```python
from build123d import *

# Parameters (mm, degrees)
SKETCH1_W           = 45.5
SKETCH1_H           = 37
BASIS_DEPTH         = 4
CUT_EXTRUDE10_DEPTH = 0.1
CUT_EXTRUDE14_DEPTH = 0.1
SKETCH10_9_R        = 5.5
SKETCH10_9_R_2      = 5.3
CUT_EXTRUDE16_DEPTH = 0.1
FILLET1_R           = 0.2


with BuildPart() as part:
    # Sketch1 → Basis (new body)
    with BuildSketch(Plane.XY):
        with Locations((22.75, 18.5)):
            Rectangle(SKETCH1_W, SKETCH1_H)
        Polygon((14.5, 39.5), (12.5, 37), (16.5, 37), align=None)
        Polygon((31, 39.5), (29, 37), (33, 37), align=None)
        Polygon((16.5, 0), (12.5, 0), (14.5, -2.5), align=None)
        Polygon((33, 0), (29, 0), (31, -2.5), align=None)
    extrude(amount=BASIS_DEPTH)

    # Sketch10 → Cut-Extrude10 (cut)
    with BuildSketch(Plane.XY.offset(4)):
        with BuildLine():
            Line((10.75, 12), (34.75, 12))
            add(Edge.make_bspline(
                [(10.75, 12), (10.75, 5), (22.75, 5), (34.75, 5), (34.75, 12)],
                knots=[0, 0, 0, 1.570796327, 1.570796327, 3.141592654, 3.141592654, 3.141592654], degree=2, weights=[1, 0.707106781, 1, 0.707106781, 1]))
        make_face()
        with BuildLine():
            Line((10.955151261, 11.8), (34.544848739, 11.8))
            add(Edge.make_bspline(
                [(34.544848739, 11.8), (34.522497462, 11.366189062), (34.337619942, 10.522792028), (33.405825268, 8.867470761), (31.220098023, 7.030241966), (27.326621533, 5.547133455), (22.75, 5.026433272), (18.173378467, 5.547133455), (14.279901977, 7.030241966), (12.094174732, 8.867470761), (11.162380058, 10.522792028), (10.977502538, 11.366189062), (10.955151261, 11.8)],
                knots=[3.171638741, 3.171638741, 3.171638741, 3.171638741, 3.364232521, 3.556826301, 3.942013861, 4.32720142, 4.71238898, 5.09757654, 5.4827641, 5.86795166, 6.06054544, 6.25313922, 6.25313922, 6.25313922, 6.25313922], degree=3))
        make_face(mode=Mode.SUBTRACT)
    extrude(amount=-CUT_EXTRUDE10_DEPTH, mode=Mode.SUBTRACT)

    # Sketch10_6 → Cut-Extrude14 (cut)
    with BuildSketch(Plane.XY.offset(4)):
        with BuildLine():
            ThreePointArc((12.125360528, 18.820696373), (13.25, 18.7), (14.374639472, 18.820696373))
            add(Edge.make_bspline(
                [(14.374639472, 18.820696373), (17.140586708, 20.492548158), (15.195293354, 23.38435682), (13.25, 26.276165482), (11.304706646, 23.38435682), (9.359413292, 20.492548158), (12.125360528, 18.820696373)],
                knots=[0.46660386, 0.46660386, 0.46660386, 2.249929722, 2.249929722, 4.033255585, 4.033255585, 5.816581447, 5.816581447, 5.816581447], degree=2, weights=[1, 0.62811894, 1, 0.62811894, 1, 0.62811894, 1]))
        make_face()
    cut_extrude14 = extrude(amount=-CUT_EXTRUDE14_DEPTH, mode=Mode.SUBTRACT)

    # Sketch10_9 → Cut-Extrude16 (cut)
    with BuildSketch(Plane.XY.offset(4)):
        with Locations((13.25, 24)):
            Circle(SKETCH10_9_R)
        with Locations((13.25, 24)):
            Circle(SKETCH10_9_R_2, mode=Mode.SUBTRACT)
    cut_extrude16 = extrude(amount=-CUT_EXTRUDE16_DEPTH, mode=Mode.SUBTRACT)

    # Mirror1: Cut-Extrude14, Cut-Extrude16 across plane
    add(cut_extrude14.mirror(Plane.ZY.offset(-22.75)), mode=Mode.SUBTRACT)
    add(cut_extrude16.mirror(Plane.ZY.offset(-22.75)), mode=Mode.SUBTRACT)

    # Fillet1
    fillet1_edges = [part.edges().sort_by_distance(p)[0] for p in [
        (10.955151261, 11.8, 3.95),
        (34.544848739, 11.8, 3.95),
        (10.75, 12, 3.95),
        (34.75, 12, 3.95),
    ]]
    fillet(fillet1_edges, radius=FILLET1_R)


solid = part.part
```
Input: part model. Units: mm. Frame: model coordinates. A direction names the side the tool comes from. Coordinates: 2 decimals unless noted, no trailing zeros. Loops run counter-clockwise (first coordinate to the right, second up) from the corner with the lowest first, then second, coordinate; pieces in that order, holes last. Notation, with made-up numbers: (44, -15.5) -> (64, -15.5) arc R21 cw to (64, 6.5) -> close; hole circle Ø1 at (-6, 76). An arc over 180 degrees is marked (long way). Use a Markdown table: item, result.
1) Cut plane A-A (z = 3.2). Return the cut outline in (x, y).
Results found:
| item | result |
|---|---|
| outline | (0, 0) -> (12.5, 0) -> (14.5, -2.5) -> (16.5, 0) -> (29, 0) -> (31, -2.5) -> (33, 0) -> (45.5, 0) -> (45.5, 37) -> (33, 37) -> (31, 39.5) -> (29, 37) -> (16.5, 37) -> (14.5, 39.5) -> (12.5, 37) -> (0, 37) -> close |
2) Material intervals for line 1 along Y through (x, z) = (25, 0.9), sorted ascending. Write a range as from..to.
Results found:
| item | result |
|---|---|
| line 1 | y = 0..37 |
3) Pull-direction query (Y, two-part tool) for faces 3 (the flat face through (39, 37, 2)), 4 (the flat face through (32, 25, 4)), 5 (the flat face through (13, 22, 3.9)); classes: released by +Y, released by -Y, zero draft, split by the parting line, or undercut.
Results found:
| item | result |
|---|---|
| face 3 | released by +Y |
| face 4 | zero draft |
| face 5 | undercut |
4) Access query for faces 1 (the flat face through (29.986, -1.233, 1.972)), 2 (the flat face through (31.986, -1.267, 1.972)). Directions: +Z, -Z, +X, -X, +Y, -Y. A direction counts if a zero-diameter tool reaches every point of the face in a straight line with its end or side. Return the directions, or none.
Results found:
| item | result |
|---|---|
| face 1 | +Z, -Z, -Y |
| face 2 | +Z, -Z, +X, -Y |
5) Cut plane C-C (x = 36). Return the cut outline in (y, z), then the cut area to 3 significant figures.
Results found:
| item | result |
|---|---|
| outline | (0, 0) -> (37, 0) -> (37, 4) -> (28.02, 4) -> (28.02, 3.9) -> (27.75, 3.9) -> (27.75, 4) -> (20.25, 4) -> (20.25, 3.9) -> (19.98, 3.9) -> (19.98, 4) -> (0, 4) -> close |
| area | 148 mm2 |
6) Cut plane B-B (x = 8.5). Return the cut outline in (y, z).
Results found:
| item | result |
|---|---|
| outline | (0, 0) -> (37, 0) -> (37, 4) -> (26.77, 4) -> (26.77, 3.9) -> (26.35, 3.9) -> (26.35, 4) -> (21.65, 4) -> (21.65, 3.9) -> (21.23, 3.9) -> (21.23, 4) -> (0, 4) -> close |
7) Contact query for flat-ended pins moving along their axis: pin 1 (1.2 mm diameter, centred on x = 22.5, z = 2, fed in from +Y); pin 2 (1.5 mm diameter, centred on x = 25, z = 1.5, fed in from -Y). Output: stop coordinate, or through.
Results found:
| item | result |
|---|---|
| pin 1 | stops at y = 37 |
| pin 2 | stops at y = 0 |
